from build123d import *

# Parameters (mm, degrees)
SKETCH1_W           = 25
SKETCH1_H           = 90
BOSS_EXTRUDE1_DEPTH = 9
SKETCH4_W           = 8
SKETCH4_H           = 71
SKETCH5_W           = 25
SKETCH5_H           = 2.4
SKETCH5_W_2         = 28
FLANGE_SLOT_DEPTH   = 8.2
SKETCH6_W           = 8.432931683
SKETCH6_H           = 8.432931683
SKETCH18_W          = 25
SKETCH18_H          = 50
SYRINGE_BAY_DEPTH   = 7
SKETCH26_W          = 38.352553791
SKETCH26_H          = 20.215566654
CUT_EXTRUDE14_DEPTH = 10
LPATTERN3_COUNT     = 2
LPATTERN3_PITCH     = 20.4
SKETCH31_R          = 1.9
CUT_EXTRUDE16_DEPTH = 4
SKETCH33_R          = 1.9
BOSS_EXTRUDE2_DEPTH = 4
FILLET1_R           = 0.4
FILLET2_R           = 0.6
CUT_EXTRUDE17_DEPTH = 10
FILLET7_R           = 1


with BuildPart() as part:
    # Sketch1 → Boss-Extrude1 (new body)
    with BuildSketch(Plane(origin=(0, 0, 0), x_dir=(1, 0, 0), z_dir=(0, 1, 0))):
        Rectangle(SKETCH1_W, SKETCH1_H)
    extrude(amount=BOSS_EXTRUDE1_DEPTH)

    # Sketch4 → Syringe Body slot (revolve, cut)
    with BuildSketch(Plane(origin=(0, 9, 0), x_dir=(1, 0, 0), z_dir=(0, 1, 0))):
        with Locations((-4, 1.3)):
            Rectangle(SKETCH4_W, SKETCH4_H)
    revolve(axis=Axis((0, 9, -36.8), (0, 0, 1)), mode=Mode.SUBTRACT)

    # Sketch5 → Flange Slot (cut)
    with BuildSketch(Plane(origin=(0, 9, 0), x_dir=(1, 0, 0), z_dir=(0, 1, 0))):
        with Locations((0, -35.367068317)):
            Rectangle(SKETCH5_W, SKETCH5_H)
        with Locations((0, -39.936134865)):
            Rectangle(SKETCH5_W_2, SKETCH5_H)
    extrude(amount=-FLANGE_SLOT_DEPTH, mode=Mode.SUBTRACT)

    # Sketch6 → Plunger Slot (revolve, cut)
    with BuildSketch(Plane(origin=(0, 9, 0), x_dir=(1, 0, 0), z_dir=(0, 1, 0))):
        with Locations((-4.216465842, -40.783534159)):
            Rectangle(SKETCH6_W, SKETCH6_H)
    revolve(axis=Axis((0, 9, 45), (0, 0, -1)), mode=Mode.SUBTRACT)

    # Sketch18 → Syringe Bay (cut)
    with BuildSketch(Plane(origin=(0, 9, 0), x_dir=(1, 0, 0), z_dir=(0, 1, 0))):
        Rectangle(SKETCH18_W, SKETCH18_H)
    extrude(amount=-SYRINGE_BAY_DEPTH, mode=Mode.SUBTRACT)

    # Sketch26 → Cut-Extrude14 (cut)
    with BuildSketch(Plane(origin=(0, 9, 0), x_dir=(1, 0, 0), z_dir=(0, 1, 0))):
        with Locations((-0.72363309, 35.107783327)):
            Rectangle(SKETCH26_W, SKETCH26_H)
    extrude(amount=-CUT_EXTRUDE14_DEPTH, mode=Mode.SUBTRACT)


with BuildPart() as lpattern3_1:
    # LPattern3: pattern copy
    add(part.part.moved(Location(Vector(1, 0, 0) * (1 * LPATTERN3_PITCH))))


with BuildPart() as part_1:
    add(part.part)

    # Sketch31 → Cut-Extrude16 (cut)
    with BuildSketch(Plane.ZY.offset(12.5)):
        with Locations((29.687280392, 2.231257616)):
            Circle(SKETCH31_R)
    extrude(amount=-CUT_EXTRUDE16_DEPTH, mode=Mode.SUBTRACT)

    # Fillet2
    # the kernel refuses this fillet: 0.6 mm, written as the material it adds along each edge
    with BuildSketch(Plane(origin=(-8.5, 2.231257616, 29.687280392), x_dir=(0, 0, 1), z_dir=(0, -1, 0))) as fillet2_piece_1:
        with BuildLine():
            CenterArc((1.9 - FILLET2_R, FILLET2_R), FILLET2_R, 270, 90)
            Line((1.9 - FILLET2_R, 0), (1.9, 0))
            Line((1.9, 0), (1.9, FILLET2_R))
        make_face()
    revolve(axis=Axis((-8.5, 2.231257616, 29.687280392), (-1, 0, 0)))
    # the kernel refuses this fillet: 0.6 mm, written as the material it takes off along each edge
    with BuildSketch(Plane(origin=(-12.5, 2.231257616, 29.687280392), x_dir=(0, 0, 1), z_dir=(0, -1, 0))) as fillet2_2_piece_1:
        with BuildLine():
            CenterArc((1.9 + FILLET2_R, -FILLET2_R), FILLET2_R, 90, 90)
            Line((1.9, -FILLET2_R), (1.9, 0))
            Line((1.9, 0), (1.9 + FILLET2_R, 0))
        make_face()
    revolve(axis=Axis((-12.5, 2.231257616, 29.687280392), (-1, 0, 0)), mode=Mode.SUBTRACT)


with BuildPart() as body_3:
    # Sketch33 → Boss-Extrude2 (new body)
    with BuildSketch(Plane(origin=(32.9, 0, 0), x_dir=(0, 0, -1), z_dir=(1, 0, 0))):
        with Locations((-29.687280392, 2.231257616)):
            Circle(SKETCH33_R)
    extrude(amount=BOSS_EXTRUDE2_DEPTH)

    # Fillet1
    fillet1_edges = [body_3.edges().sort_by_distance(p)[0] for p in [
        (32.9, 2.231257616, 31.587280392),
        (36.9, 2.231257616, 31.587280392),
    ]]
    fillet(fillet1_edges, radius=FILLET1_R)


with BuildPart() as cut_extrude17_tool:
    # Sketch35 → Cut-Extrude17 (new body)
    with BuildSketch(Plane(origin=(0, 2, 0), x_dir=(1, 0, 0), z_dir=(0, 1, 0))):
        with BuildLine():
            Line((-7.572519934, 18.75), (-7.572519934, -18.75))
            ThreePointArc((-7.572519934, -18.75), (-14, -25.177480066), (-20.427480066, -18.75))
            Line((-20.427480066, -18.75), (-20.427480066, 18.75))
            ThreePointArc((-20.427480066, 18.75), (-14, 25.177480066), (-7.572519934, 18.75))
        make_face()
        with BuildLine():
            Line((15.038012539, 25.284497927), (15.038012539, 10.435091669))
            ThreePointArc((15.038012539, 10.435091669), (10.258664257, 12.127791533), (5.538012539, 10.277696889))
            Line((5.538012539, 10.277696889), (5.538012539, 25.284497927))
            ThreePointArc((5.538012539, 25.284497927), (10.288012539, 30.034497927), (15.038012539, 25.284497927))
        make_face()
        with BuildLine():
            Line((28.019587368, 18.885486869), (28.305082347, -18.61342635))
            ThreePointArc((28.305082347, -18.61342635), (34.781309827, -24.991786455), (41.159669932, -18.515558975))
            Line((41.159669932, -18.515558975), (40.874174953, 18.983354244))
            ThreePointArc((40.874174953, 18.983354244), (34.397947473, 25.361714349), (28.019587368, 18.885486869))
        make_face()
        with BuildLine():
            Line((15.038012539, -0.688026199), (15.038012539, -18.75))
            ThreePointArc((15.038012539, -18.75), (10.288012539, -23.5), (5.538012539, -18.75))
            Line((5.538012539, -18.75), (5.538012539, -0.530631419))
            ThreePointArc((5.538012539, -0.530631419), (10.258664257, -2.380726063), (15.038012539, -0.688026199))
        make_face()
    extrude(amount=-CUT_EXTRUDE17_DEPTH)


with BuildPart() as part_2:
    add(part_1.part)

    # Cut-Extrude17: cut by cut_extrude17_tool
    add(cut_extrude17_tool.part, mode=Mode.SUBTRACT)


with BuildPart() as lpattern3_1_1:
    add(lpattern3_1.part)

    # Cut-Extrude17: cut by cut_extrude17_tool
    add(cut_extrude17_tool.part, mode=Mode.SUBTRACT)

    # Combine2: union part, body 3
    add(part_2.part)
    add(body_3.part)

    # Fillet7
    fillet7_edges = [lpattern3_1_1.edges().sort_by_distance(p)[0] for p in [
        (7.9, 9, 29.583534158),
        (10.2, 9, 25),
        (30.65, 9, 25),
        (10.2, 9, 45),
        (32.9, 9, 37.651601591),
        (32.9, 9, 29.583534158),
        (7.9, 9, 37.651601591),
        (7.9, 9, 43.068067433),
        (10.2, 9, 41.136134865),
        (30.866465842, 9, 38.736134865),
        (-10.25, 9, 34.167068317),
        (12.5, 9, 37.651601591),
        (12.5, 9, 43.068067433),
        (-8.432931683, 9, 37.651601591),
        (-8.432931683, 9, 43.068067433),
        (-12.5, 9, 29.583534158),
        (-8, 9, 29.583534158),
        (12.5, 9, 29.583534158),
        (-12.5, 9, 37.651601591),
        (-12.5, 9, 43.068067433),
        (-10.466465842, 9, 45),
        (-10.466465842, 9, 38.736134865),
        (-10.466465842, 9, 36.567068317),
        (-10.466465842, 9, 41.136134865),
        (-10.25, 9, 25),
        (10.2, 9, 34.167068317),
        (10.2, 9, 36.567068317),
        (30.65, 9, 34.167068317),
        (32.9, 9, 43.068067433),
        (10.2, 9, 38.736134865),
        (30.866465842, 9, 41.136134865),
        (30.866465842, 9, 36.567068317),
        (30.866465842, 9, 45),
        (28.832931683, 9, 37.651601591),
        (28.832931683, 9, 43.068067433),
        (28.4, 9, 29.583534158),
    ]]
    fillet(fillet7_edges, radius=FILLET7_R)


solid = lpattern3_1_1.part
Geometry: final body of the model. Coordinates: model frame, mm. A direction names the side the tool comes from. Round coordinates to 2 decimals unless told otherwise and drop trailing zeros. Order: outer loops, then holes, each group sorted by start corner. A loop starts at its lowest first (then second) coordinate and runs counter-clockwise, first axis right, second up. Notation, with made-up numbers: (88, -5.75) - (117, -5.75) arc R21 ccw to (117, 26.25) - close; hole circle Ø8 at (82, 18). An arc over 180 degrees is marked (long way). Write each question's results on one line, items separated by ' | '.
Item 1: Reachability of faces 5 (the flat face through (10, 2, 0)), 6 (the flat face through (10, 0.8, 40)), 7 (the flat face through (5.538, 1, -18)), 8 (the cylindrical face through (-8.99, 1.014, -22.776)) from +Z, -Z, +X, -X, +Y, -Y: full face, straight path, thin tool, end or side. Return the list, or none.
Completed:
face 5: -Z, +X, -X, +Y | face 6: +X, -X, +Y | face 7: -Z, +Y, -Y | face 8: -X, +Y, -Y
Item 2: First-contact query: pin 1 Ø9.5 at (x, z) = (27, 2.5) entering from +Y; pin 2 Ø3 at (y, z) = (2.23, 29.69) entering from -X; pin 3 Ø2 at (x, y) = (27, 5) entering from -Z. Flat tips, straight axial feed; report the tip coordinate or a pass-through.
Completed:
pin 1: y = 2 | pin 2: x = -8.54 | pin 3: z = 25
Item 3: Section A-A, the plane x = 13.5. Return the cut outline in (y, z), and give its area (3 significant figures).
Completed:
outline: (0, -11.42) - (2, -11.42) - (2, 1.68) - (0, 1.68) - close; (0, 22.25) - (2, 22.25) - (2, 25) - (4.95, 25) - (4.95, 34.17) - (0.8, 34.17) - (0.8, 36.57) - (4.15, 36.57) - (4.15, 38.74) - (0.8, 38.74) - (0.8, 41.14) - (4.15, 41.14) - (4.15, 45) - (0, 45) - close | area: 106 mm^2
Item 4: Section B-B, the plane x = 1. Return the cut outline in (y, z), and give its area (3 significant figures).
Completed:
outline: (0, -25) - (1.06, -25) - (1.06, 34.17) - (0.8, 34.17) - (0.8, 36.57) - (0.63, 36.57) - (0.63, 45) - (0, 45) - close | area: 70.1 mm^2
Item 5: Mould query, pull axis Z, two halves, no side actions, for faces 1 (the flat face through (10, 4, 34.167)), 2 (the cylindrical face through (34.88, 1.08, 31.2)), 3 (the flat face through (29, 5, 25)), 4 (the flat face through (-10, 9, 30)). Classes: pulls with the +Z half, pulls with the -Z half, needs draft (parallel to the pull), parting line crosses it, or undercut.
Completed:
face 1: undercut | face 2: parting line crosses it | face 3: pulls with the -Z half | face 4: needs draft
Item 6: Material intervals for line 1 along Z through (x, y) = (-5, 1.5); line 2 along X through (y, z) = (5.25, 42.5); line 3 along Z through (x, y) = (27.5, 4.75), sorted ascending. Write a range as [from, to].
Completed:
line 1: [-25, 34.17], [36.57, 38.74], [41.14, 45] | line 2: [-12.5, -7.55], [7.55, 12.85], [27.95, 32.9] | line 3: [25, 34.17]
